Design review of the part built by this model. Coordinates are the model's own, in mm. Give positions to 0.01 mm unless a question says otherwise; leave off trailing zeros. Write each loop counter-clockwise with the first axis right and the second up, starting at its lowest first coordinate (ties: lowest second). Pieces come first, ordered by that corner, then holes. Notation, with made-up numbers: M -10.75,59 L 42.25,59 A27 ccw 42.25,98 Z; hole C 70,57.25 d7. An arc over 180 degrees is marked long. Use one line per item in the form item = value. Start each with the question number.
from build123d import *

# Parameters (mm, degrees)
SKETCH1_R           = 49.704747918
SKETCH1_R_2         = 37.896378772
BOSS_EXTRUDE1_DEPTH = 304.8
BOSS_EXTRUDE2_START = 25.4
SKETCH2_R           = 49.704747918
BOSS_EXTRUDE2_DEPTH = 25.4
BOSS_EXTRUDE3_START = -25.4
BOSS_EXTRUDE3_DEPTH = 25.4


with BuildPart() as part:
    # Sketch1 → Boss-Extrude1 (new body)
    with BuildSketch(Plane.XY):
        with Locations(Location((0, 0, 0), (0, 0, 180))):
            Circle(SKETCH1_R)
        with Locations(Location((0, 0, 0), (0, 0, 180))):
            Circle(SKETCH1_R_2, mode=Mode.SUBTRACT)
    extrude(amount=BOSS_EXTRUDE1_DEPTH)

    # Sketch2 → Boss-Extrude2 (add)
    with BuildSketch(Plane(origin=(0, 0, 0), x_dir=(-1, 0, 0), z_dir=(0, 0, -1)).offset(BOSS_EXTRUDE2_START)):
        Circle(SKETCH2_R)
    extrude(amount=-BOSS_EXTRUDE2_DEPTH)

    # Sketch3 → Boss-Extrude3 (add)
    with BuildSketch(Plane.XY.offset(304.8).offset(BOSS_EXTRUDE3_START)):
        with BuildLine():
            ThreePointArc((37.896378772, 0), (37.700998174, 3.843209698), (37.116871006, 7.64679088))
            Line((37.116871006, 7.64679088), (-37.894810184, 0.344797316))
            ThreePointArc((-37.894810184, 0.344797316), (-0.172400442, -37.895986623), (37.896378772, 0))
        make_face()
    extrude(amount=BOSS_EXTRUDE3_DEPTH)


solid = part.part
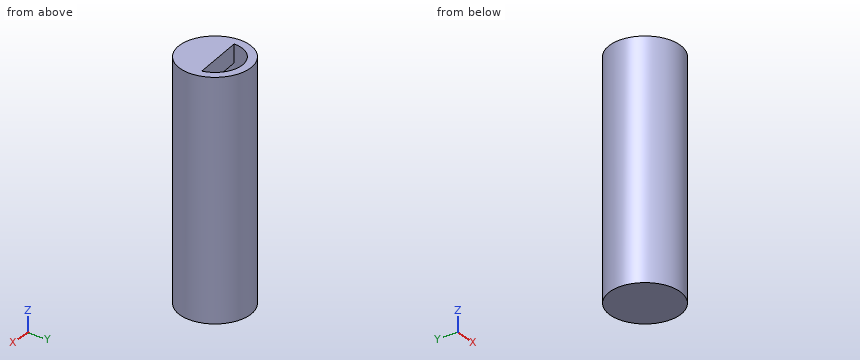
1. We need section A-A (y = -3). State the section outline as (x, z) points.
2. We need section C-C (x = 0.5). State the section outline as (y, z) points.
3. We need section D-D (y = -34). State the section outline as (x, z) points.
4. Clearance check with flat-ended pins moving along their axes: pin 1 Ø5 at (x, z) = (37.5, 170.5) entering from +Y; pin 2 Ø10 at (x, z) = (-18.5, 176) entering from -Y; pin 3 Ø3 at (y, z) = (-9.5, 172.5) entering from -X. State where each tip first meets the part, or that it passes through.
5. We need section B-B (z = 195). State the section outline as (x, y) points.
6. To check wall thickness, follow L1, parallel to Y at x = 0, z = 230.5; L2, parallel to Z at x = 34, y = -6.5. State the ranges of each line that lie inside material, in increasing order.
Answer block:
q1.outline = M -49.61,-25.4 L 49.61,-25.4 L 49.61,304.8 L -49.61,304.8 Z; hole M -37.78,0 L 37.78,0 L 37.78,279.4 L -37.78,279.4 Z
q2.outline = M -49.7,-25.4 L 49.7,-25.4 L 49.7,304.8 L 37.89,304.8 L 37.89,0 L -37.89,0 L -37.89,279.4 L 4.08,279.4 L 4.08,304.8 L -49.7,304.8 Z
q3.outline = M -36.26,-25.4 L 36.26,-25.4 L 36.26,304.8 L -36.26,304.8 Z; hole M -16.74,0 L 16.74,0 L 16.74,279.4 L -16.74,279.4 Z
q4.pin_1 = 35.29
q4.pin_2 = -47.84
q4.pin_3 = -49.06
q5.outline = C 0,0 d99.41; hole C 0,0 d75.79
q6.L1 = -49.7 to -37.9, 37.9 to 49.7
q6.L2 = -25.4 to 0, 279.4 to 304.8
